Autodesk Inventor part; units mm, degrees
ref_plane "YZ Plane" through (0, 0, 0) normal (1, 0, 0) x (0, 1, 0)
ref_plane "XZ Plane" through (0, 0, 0) normal (0, 1, 0) x (-1, 0, 0)
ref_plane "XY Plane" through (0, 0, 0) normal (0, 0, 1) x (1, 0, 0)
sketch "Esquisse1" plane through (0, 0, 0) normal (0, 0, 1) x (1, 0, 0)
  line L0 (-21.137, 18.1163) -> (26.863, 18.1163)
  line L1 (26.863, 18.1163) -> (26.863, -46.8837)
  line L2 (26.863, -46.8837) -> (-21.137, -46.8837)
  line L3 (-21.137, -46.8837) -> (-21.137, 18.1163)
  point P0 (0, 0)
  dimension "d0" = 48
  dimension "d1" = 65
extrude "Extrusion1" add sketch "Esquisse1" along normal blind 6
sketch "Esquisse2" plane through (0, 0, 6) normal (0, 0, 1) x (1, 0, 0)
  line L0 (-18.137, -40.8837) -> (-15.137, -40.8837)
  line L1 (-15.137, -40.8837) -> (-15.137, -43.8837)
  line L2 (-15.137, -43.8837) -> (-18.137, -43.8837)
  line L3 (-18.137, -43.8837) -> (-18.137, -40.8837)
  line L4 (20.863, -40.8837) -> (23.863, -40.8837)
  line L5 (23.863, -40.8837) -> (23.863, -43.8837)
  line L6 (23.863, -43.8837) -> (20.863, -43.8837)
  line L7 (20.863, -43.8837) -> (20.863, -40.8837)
  line L8 (23.863, 12.1163) -> (20.863, 12.1163)
  line L9 (20.863, 12.1163) -> (20.863, 15.1163)
  line L10 (20.863, 15.1163) -> (23.863, 15.1163)
  line L11 (23.863, 15.1163) -> (23.863, 12.1163)
  line L12 (-15.137, 12.1163) -> (-18.137, 12.1163)
  line L13 (-18.137, 12.1163) -> (-18.137, 15.1163)
  line L14 (-18.137, 15.1163) -> (-15.137, 15.1163)
  line L15 (-15.137, 15.1163) -> (-15.137, 12.1163)
  line L16 (26.863, 18.1163) -> (-21.137, 18.1163)
  line L17 (-21.137, 18.1163) -> (-21.137, -46.8837)
  line L18 (26.863, -46.8837) -> (26.863, 18.1163)
  line L19 (-21.137, -46.8837) -> (26.863, -46.8837)
  point P0 (0, 0)
  dimension "d4" = 3
  dimension "d5" = 3
  dimension "d6" = 3
  dimension "d7" = 3
  dimension "d8" = 3
  dimension "d9" = 3
  dimension "d10" = 3
  dimension "d11" = 3
  dimension "d12" = 3
  dimension "d13" = 3
  dimension "d14" = 3
  dimension "d15" = 3
  dimension "d16" = 3
  dimension "d17" = 3
  dimension "d18" = 3
extrude "Extrusion2" cut sketch "Esquisse2" against normal blind 2.5 contours L0 L1 L2 L3 | L4 L5 L6 L7 | L8 L9 L10 L11 | L12 L13 L14 L15
sketch "Esquisse4" plane through (0, 0, 0) normal (0, 0, -1) x (-1, 0, 0)
  line L0 (-24.863, -1.8837) -> (19.137, -1.8837)
  line L1 (19.137, -1.8837) -> (19.137, -11.8837)
  line L2 (19.137, -11.8837) -> (-24.863, -11.8837)
  line L3 (-24.863, -11.8837) -> (-24.863, -1.8837)
  line L4 (-24.863, -16.8837) -> (19.137, -16.8837)
  line L5 (19.137, -16.8837) -> (19.137, -26.8837)
  line L6 (19.137, -26.8837) -> (-24.863, -26.8837)
  line L7 (-24.863, -26.8837) -> (-24.863, -16.8837)
  line L8 (-24.863, -31.8837) -> (19.137, -31.8837)
  line L9 (19.137, -31.8837) -> (19.137, -41.8837)
  line L10 (19.137, -41.8837) -> (-24.863, -41.8837)
  line L11 (-24.863, -41.8837) -> (-24.863, -31.8837)
  line L12 (-26.863, -46.8837) -> (-26.863, 18.1163)
  line L13 (21.137, 18.1163) -> (21.137, -46.8837)
  line L14 (-24.863, 13.1163) -> (19.137, 13.1163)
  line L15 (19.137, 13.1163) -> (19.137, 3.1163)
  line L16 (19.137, 3.1163) -> (-24.863, 3.1163)
  line L17 (-24.863, 3.1163) -> (-24.863, 13.1163)
  point P0 (0, 0)
  point P1 (-20.863, 12.1163)
  dimension "d39" = 10
  dimension "d40" = 5
  dimension "d41" = 10
  dimension "d42" = 5
  dimension "d43" = 10
  dimension "d44" = 44
  dimension "d45" = 2
  dimension "d46" = 44
  dimension "d47" = 2
  dimension "d48" = 44
  dimension "d49" = 2
  dimension "d52" = 5
  dimension "d53" = 10
  dimension "d54" = 2
  dimension "d57" = 44
extrude "Extrusion4" cut sketch "Esquisse4" against normal blind 1
fillet "Congé2" radius 0.5 16 edges at (-16.637, 12.1163, 3.5) (-15.137, 13.6163, 3.5) (-16.637, 15.1163, 3.5) (-18.137, 13.6163, 3.5) (22.363, 15.1163, 3.5) (20.863, 13.6163, 3.5) (22.363, 12.1163, 3.5) (23.863, 13.6163, 3.5) (-16.637, -43.8837, 3.5) (-15.137, -42.3837, 3.5) (-18.137, -42.3837, 3.5) (-16.637, -40.8837, 3.5) (20.863, -42.3837, 3.5) (22.363, -40.8837, 3.5) (22.363, -43.8837, 3.5) (23.863, -42.3837, 3.5)
properties part number "pièce_mobile_station"
Model file for the job. Use its own axes, mm. A direction names the side the tool comes from. Round coordinates to 2 decimals unless told otherwise and drop trailing zeros. Order: outer loops, then holes, each group sorted by start corner. A loop starts at its lowest first (then second) coordinate and runs counter-clockwise, first axis right, second up.
(1) Drill centre lines: line 1 (X direction, y = 13.5, z = 4.5); line 2 (Y direction, x = -0.5, z = 0.9); line 3 (Z direction, x = -15, y = -10). Where is each one in solid material? Low to high.
(2) Pull direction Y, two halves, no side cores. Call faces 1 (the face through (3, -46.884, 3)), 2 (the face through (3, -14, 6)), 3 (the face through (3, 8, 1)): released by +Y, released by -Y, zero draft, split by the parting line, or undercut.
(3) Band-saw the part on B-B (y = 5.5). List the corners of the cut face in (x, z), then the cut area to 3 significant figures.
(4) Pin check, flat tips, straight feed: pin 1 (2 mm diameter, centred on x = -16.5, y = -42.5, fed in from +Z); pin 2 (4 mm diameter, centred on x = 11, y = -23.5, fed in from -Z). Stop position of each tip, or through.
(5) Band-saw the part on A-A (x = -4.5). List the corners of the cut face in (y, z), then the cut area to 3 significant figures.
(6) 3-axis set-ups, long thin cutter, end or side, ignore diameter. For faces 4 (the face through (26.863, -14, 3)), 5 (the face through (23.863, -42, 5)), 6 (the face through (3, -37, 1)): which of +Z, -Z, +X, -X, +Y, -Y reach the whole face in a straight line?
Verdict:
1. line 1: x = -21.14 to -18.14, -15.14 to 20.86, 23.86 to 26.86
1. line 2: y = -46.88 to -41.88, -31.88 to -26.88, -16.88 to -11.88, -1.88 to 3.12, 13.12 to 18.12
1. line 3: z = 1 to 6
2. face 1: released by -Y
2. face 2: zero draft
2. face 3: undercut
3. outline: (-21.14, 0) - (-19.14, 0) - (-19.14, 1) - (24.86, 1) - (24.86, 0) - (26.86, 0) - (26.86, 6) - (-21.14, 6) - close
3. area: 244 mm2
4. pin 1: stops at z = 3.52
4. pin 2: stops at z = 1
5. outline: (-46.88, 0) - (-41.88, 0) - (-41.88, 1) - (-31.88, 1) - (-31.88, 0) - (-26.88, 0) - (-26.88, 1) - (-16.88, 1) - (-16.88, 0) - (-11.88, 0) - (-11.88, 1) - (-1.88, 1) - (-1.88, 0) - (3.12, 0) - (3.12, 1) - (13.12, 1) - (13.12, 0) - (18.12, 0) - (18.12, 6) - (-46.88, 6) - close
5. area: 350 mm2
6. face 4: +Z, -Z, +X, +Y, -Y
6. face 5: +Z
6. face 6: -Z
